Here's the drawing with two shaded views (mm, measured from the low corner). I have some questions. A direction names the side the tool comes from. Round coordinates to 2 decimals unless told otherwise and drop trailing zeros. Order: outer loops, then holes, each group sorted by start corner. A loop starts at its lowest first (then second) coordinate and runs counter-clockwise, first axis right, second up.
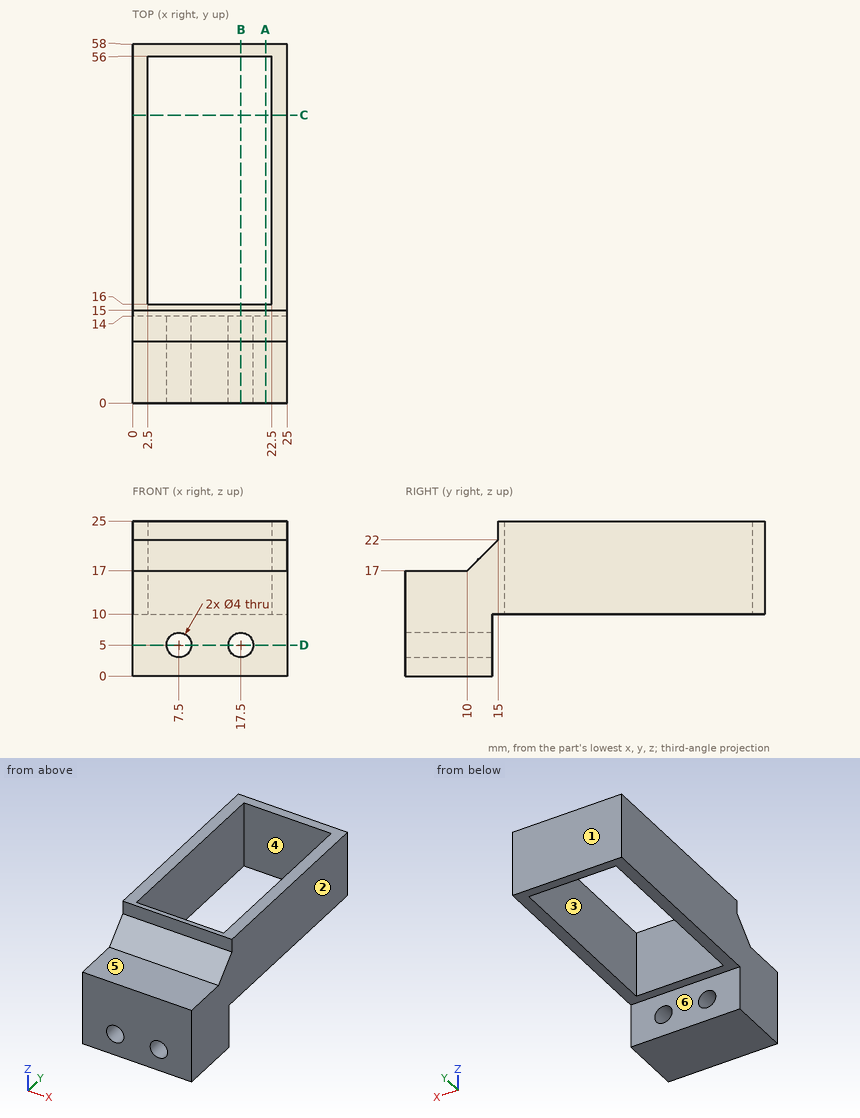
1. On a 3-axis mill with a long thin cutter (end or side, diameter ignored), from which of +Z, -Z, +X, -X, +Y, -Y can I reach the whole of each face in a straight line? I mean the marked faces 4, 5 and 6. Say none if no direction works.
Evaluation:
face 4: +Z, -Z
face 5: +Z, +X, -X, -Y
face 6: -Z, +X, -X, +Y
2. I need wall thicknesses on probe 1 along X at (y, z) = (10.5, 5); probe 2 along Y at (x, z) = (2.75, 23.25); probe 3 along Y at (x, z) = (12.75, 12). Which ranges of each line are inside material? Lowest first, please.
Evaluation:
probe 1: x = 0 to 5.5, 9.5 to 15.5, 19.5 to 25
probe 2: y = 15 to 16, 56 to 58
probe 3: y = 0 to 16, 56 to 58
3. If we section it at A-A, the plane x = 21.5: Write out the boundary of the cut face in (y, z), and give its area (4 significant figures).
Evaluation:
outline: (0, 0) - (14, 0) - (14, 10) - (16, 10) - (16, 25) - (15, 25) - (15, 22) - (10, 17) - (0, 17) - close; (56, 10) - (58, 10) - (58, 25) - (56, 25) - close
area: 302.5 mm2
4. If we mould it in two halves opening along X, with no side actions, what happens to the marked faces 1, 2 and 3? For each: released by +X, released by -X, zero draft, split by the parting line, or undercut.
Evaluation:
face 1: zero draft
face 2: released by +X
face 3: undercut
5. If we section it at B-B, the plane x = 17.5: Write out the boundary of the cut face in (y, z).
Evaluation:
outline: (0, 0) - (14, 0) - (14, 3) - (0, 3) - close; (0, 7) - (14, 7) - (14, 10) - (16, 10) - (16, 25) - (15, 25) - (15, 22) - (10, 17) - (0, 17) - close; (56, 10) - (58, 10) - (58, 25) - (56, 25) - close
6. If we section it at C-C, the plane y = 46.5: Write out the boundary of the cut face in (x, z).
Evaluation:
outline: (0, 10) - (2.5, 10) - (2.5, 25) - (0, 25) - close; (22.5, 10) - (25, 10) - (25, 25) - (22.5, 25) - close
7. I'm going to push flat-ended pins straight in: P1, Ø0.9, axis at x = 16, z = 23.5, coming from the -Y side; P2, Ø3, axis at x = 6.5, y = 5, coming from the +Z side; P3, Ø3, axis at x = 2.5, y = 10.5, coming from the +Z side. Where does each tip first touch, or does it pass through?
Evaluation:
P1: stops at y = 15
P2: stops at z = 17
P3: stops at z = 19
8. If we section it at D-D, the plane z = 5: Write out the boundary of the cut face in (x, y), and give its area (3 significant figures).
Evaluation:
outline: (0, 0) - (5.5, 0) - (5.5, 14) - (0, 14) - close; (9.5, 0) - (15.5, 0) - (15.5, 14) - (9.5, 14) - close; (19.5, 0) - (25, 0) - (25, 14) - (19.5, 14) - close
area: 238 mm2
